Here's how the part is built. I have some questions about the finished solid (model axes, mm). A direction names the side the tool comes from. Give positions to 0.01 mm unless a question says otherwise; leave off trailing zeros. Write each loop counter-clockwise with the first axis right and the second up, starting at its lowest first coordinate (ties: lowest second). Pieces come first, ordered by that corner, then holes. Notation, with made-up numbers: (69.5, -26) - (92.5, -26) arc R26 cw to (92.5, 5) - close; hole circle Ø5 at (80.5, 44.5). An arc over 180 degrees is marked (long way). One line per item, written item: value. Start each with the question number.
1) Imagine slicing it at A-A on x = 0. Write out the boundary of the cut face in (y, z), plus the area to 3 significant figures.
2) On a 3-axis mill with a long thin cutter (end or side, diameter ignored), from which of +Z, -Z, +X, -X, +Y, -Y can I reach the whole of each face in a straight line? I mean faces 1 (the flat face through (5.525, -3.131, 8.609)), 2 (the cylindrical face through (-0.2, 25.4, 11)), 3 (the flat face through (15.52, 37.47, 0.07)). Say none if no direction works.
3) Imagine slicing it at B-B on z = 7. Write out the boundary of the cut face in (x, y).
4) We'd pull the mould along X, two halves only. Please class faces 4 (the cylindrical face through (-26.89, -26.99, -0.07)), 5 (the cylindrical face through (-37.275, 21.612, 0.067)), 6 (the cylindrical face through (21.612, 37.275, 0.067)): +X half, -X half, draft (parallel to the pull), parting line (faces both ways), or undercut.
5) Please list where these lines run through material, in increasing order: L1, parallel to Y at x = 0, z = -2.8; L2, parallel to X at y = 25, z = 0.5; L3, parallel to X at y = 0, z = 7.25. Write a range as [from, to].
6) I'm going to push flat-ended pins straight in: P1, Ø2, axis at x = 0, z = 8.5, coming from the -Y side; P2, Ø10, axis at x = 10, z = 11, coming from the -Y side; P3, Ø6, axis at x = -1, z = 6, coming from the +Y side. Where does each tip first touch, or does it pass through?
7) Imagine slicing it at D-D on x = 17.5. Write out the boundary of the cut face in (y, z).
8) Imagine slicing it at C-C on y = -20.5. Write out the boundary of the cut face in (x, z).
Autodesk Inventor part; units mm, degrees
ref_plane "YZ Plane" through (0, 0, 0) normal (1, 0, 0) x (0, 1, 0)
ref_plane "XZ Plane" through (0, 0, 0) normal (0, 1, 0) x (-1, 0, 0)
ref_plane "XY Plane" through (0, 0, 0) normal (0, 0, 1) x (1, 0, 0)
sketch "Sketch1" plane through (0, 0, 0) normal (0, 0, 1) x (1, 0, 0)
  circle A0 centre (0, 0) radius 38.1
  dimension "d0" = 76.2
extrude "Extrusion1" add sketch "Sketch1" along normal mid plane 9.525
sketch "Sketch8" plane through (0, 0, 4.7625) normal (0, 0, 1) x (1, 0, 0)
  arc A0 (5.624, 42.7187) -> (-5.624, 42.7187) centre (0, 0) ccw
  circle A1 centre (0, 0) radius 38.1
  line L0 (4.973, 37.774) -> (5.624, 42.7187)
  line L1 (-4.973, 37.774) -> (-5.624, 42.7187)
  line L2 (0, 0) -> (0, 43.0873) construction
  arc A2 (4.973, 37.774) -> (-4.973, 37.774) centre (0, 0) ccw
  dimension "d40" = 4.9873
  dimension "d41" = 15
  dimension "d42" = 7.5
extrude "Extrusion9" add sketch "Sketch8" against normal blind 9.525 contours L0 A1 L1 A0
pattern_circular "Circular Pattern4" count 12 over 360 about axis through (0, 0, -10) along (0, 0, 1) of "Extrusion9"
sketch "Sketch10" plane through (0, 0, 4.7625) normal (0, 0, 1) x (1, 0, 0)
  line L0 (7.3323, 0) -> (3.6662, -6.35)
  line L1 (3.6662, -6.35) -> (-3.6662, -6.35)
  line L2 (-3.6662, -6.35) -> (-7.3323, 0)
  line L3 (-7.3323, 0) -> (-3.6662, 6.35)
  line L4 (-3.6662, 6.35) -> (3.6662, 6.35)
  line L5 (3.6662, 6.35) -> (7.3323, 0)
  point P0 (0, 0)
  point P1 (0, 0)
  dimension "d55" = 12.7
extrude "Extrusion11" cut sketch "Sketch10" against normal through all
sketch "Sketch11" plane through (0, 0, -4.7625) normal (0, 0, -1) x (-1, 0, 0)
  circle A0 centre (0, 0) radius 25.4
  dimension "d58" = 50.8
extrude "Extrusion12" cut sketch "Sketch11" against normal blind 4.7625
sketch "Sketch12" plane through (0, 0, 4.7625) normal (0, 0, 1) x (1, 0, 0)
  line L0 (7.3323, 0) -> (3.6662, -6.35)
  line L1 (3.6662, -6.35) -> (-3.6662, -6.35)
  line L2 (-3.6662, -6.35) -> (-7.3323, 0)
  line L3 (-7.3323, 0) -> (-3.6662, 6.35)
  line L4 (-3.6662, 6.35) -> (3.6662, 6.35)
  line L5 (3.6662, 6.35) -> (7.3323, 0)
  circle A0 centre (0, 0) radius 25.4
  line L6 (-12.7, 21.997) -> (-12.7, -21.997)
  line L7 (12.7, 21.997) -> (12.7, -21.997)
  arc A1 (12.7, 21.997) -> (-12.7, 21.997) centre (0, 0) ccw
  arc A2 (-12.7, -21.997) -> (12.7, -21.997) centre (0, 0) ccw
  dimension "d61" = 12.7
  dimension "d65" = 25.4
extrude "Extrusion14" add sketch "Sketch12" along normal blind 12.7 contours L7 A0 L6
equation "\"d0\" = externalDiameter"
equation "\"d40\" = depthOfExternalSpline"
equation "\"d55\" = hexSize"
equation "\"internalDiameter\" = 50.8"
equation "\"externalDiameter\" = 76.2"
equation "\"pi\" = 3.141593"
equation "\"depthOfInternalSpline\" = 0.5 * widthOfInternalSpline"
equation "\"depthOfExternalSpline\" = 0.5 * widthOfExternalSpline"
equation "\"thickness\" = 9.525"
equation "\"hexSize\" = 12.7"
properties part number "gearLock" material "PC/ABS Plastic"
Numbers:
1. outline: (-43.09, -4.76) - (-25.4, -4.76) - (-25.4, 0) - (-6.35, 0) - (-6.35, 17.46) - (-25.4, 17.46) - (-25.4, 4.76) - (-43.09, 4.76) - close; (6.35, 0) - (25.4, 0) - (25.4, -4.76) - (43.09, -4.76) - (43.09, 4.76) - (25.4, 4.76) - (25.4, 17.46) - (6.35, 17.46) - close
1. area: 1,000 mm^2
2. face 1: +Z, -Z
2. face 2: +Z, +Y
2. face 3: +Z, -Z, +Y
3. outline: (-12.7, -22) arc R25.4 ccw to (12.7, -22) - (12.7, 22) arc R25.4 ccw to (-12.7, 22) - close; hole (-7.33, 0) - (-3.67, -6.35) - (3.67, -6.35) - (7.33, 0) - (3.67, 6.35) - (-3.67, 6.35) - close
4. face 4: undercut
4. face 5: -X half
4. face 6: +X half
5. L1: [-43.09, -25.4], [25.4, 43.09]
5. L2: [-35.09, -32.58], [-28.75, 28.75], [32.58, 35.09]
5. L3: [-12.7, -7.33], [7.33, 12.7]
6. P1: y = -25.4
6. P2: y = -24.9
6. P3: y = 43.09
7. outline: (-39.37, -4.76) - (-18.41, -4.76) - (-18.41, 0) - (18.41, 0) - (18.41, -4.76) - (39.37, -4.76) - (39.37, 4.76) - (-39.37, 4.76) - close
8. outline: (-37.9, -4.76) - (-15, -4.76) - (-15, 0) - (15, 0) - (15, -4.76) - (37.9, -4.76) - (37.9, 4.76) - (12.7, 4.76) - (12.7, 17.46) - (-12.7, 17.46) - (-12.7, 4.76) - (-37.9, 4.76) - close
